Read the model definition and answer for the solid it produces. Units are mm, in the model's axes. Face numbers are marked on the shaded views. A direction names the side the tool comes from. Coordinates: 2 decimals unless noted, no trailing zeros. Write each loop counter-clockwise with the first axis right and the second up, starting at its lowest first coordinate (ties: lowest second). Pieces come first, ordered by that corner, then holes. Notation, with made-up numbers: (13.25, 12.5) -> (42.25, 12.5) arc R6 cw to (42.25, 21.5) -> close; hole circle Ø6 at (-13.5, -13.75). An arc over 180 degrees is marked (long way). Answer as a JSON object with one key per item and string values. Group by question number.
(1) Straight lines are drawn through the part: L1, parallel to Z at x = -51.4, y = -0.8; L2, parallel to X at y = -14, z = 2; L3, parallel to Z at x = 53, y = -2.5. For each, find the intervals that lie inside material, in ascending order.
(2) Flat-ended cylindrical pins translate along their axes: P1, Ø1, axis at x = -0.5, y = -8.5, coming from the -Z side; P2, Ø3, axis at x = -51.4, z = 8.2, coming from the -Y side; P3, Ø1.5, axis at x = 0, z = -8.2, coming from the +Y side. Find the tip coordinate at first contact, or state that the pin passes through.
(3) For a pull along X with two mould halves and no side action, classify the marked faces 1, 2, 3 and 4 as +X half, -X half, draft (parallel to the pull), parting line (faces both ways), or undercut.
(4) Find section A-A (x = 0). Give the vertices of the cut face in (y, z), then the cut area to 3 significant figures.
(5) Find section D-D (z = 0). Give the vertices of the cut face in (x, y).
(6) Find section B-B (y = -21.5). Give the vertices of the cut face in (x, z).
(7) Which of the six approach directions +Z, -Z, +X, -X, +Y, -Y give full straight-line access (tool end or side, diameter ignored) to the marked faces 5 and 6?
(8) Find section C-C (z = -8.2). Give the vertices of the cut face in (x, y).
from build123d import *

# Parameters (mm, degrees)
F0_W     = 124
F0_H     = 32
F0_R     = 1.25
F0_R_2   = 5.2
F0_R_3   = 4.95
F1_DEPTH = 3
F0_H_2   = 3
F2_DEPTH = 50
F5_DEPTH = 3
F6_DEPTH = 3


with BuildPart() as f1:
    # F0 (on Front) → F1 (new body)
    with BuildSketch(Plane.XZ):
        with Locations((0, 1)):
            Rectangle(F0_W, F0_H)
        with Locations((-51.4, -8.2)):
            Circle(F0_R, mode=Mode.SUBTRACT)
        with Locations((-51.4, 0)):
            Circle(F0_R_2, mode=Mode.SUBTRACT)
        with Locations((-8.2, 0)):
            Circle(F0_R, mode=Mode.SUBTRACT)
        with Locations((0, -8.2)):
            Circle(F0_R, mode=Mode.SUBTRACT)
        with Locations((51.4, -8.2)):
            Circle(F0_R, mode=Mode.SUBTRACT)
        Circle(F0_R_3, mode=Mode.SUBTRACT)
        with Locations((8.2, 0)):
            Circle(F0_R, mode=Mode.SUBTRACT)
        with Locations((51.4, 0)):
            Circle(F0_R_2, mode=Mode.SUBTRACT)
        with Locations((-51.4, 8.2)):
            Circle(F0_R, mode=Mode.SUBTRACT)
        with Locations((0, 8.2)):
            Circle(F0_R, mode=Mode.SUBTRACT)
        with Locations((51.4, 8.2)):
            Circle(F0_R, mode=Mode.SUBTRACT)
    extrude(amount=F1_DEPTH)

    # F0 (on Front) → F2 (join)
    with BuildSketch(Plane.XZ):
        with Locations((0, 18.5)):
            Rectangle(F0_W, F0_H_2)
    extrude(amount=F2_DEPTH)

    # F4 (on face) → F5 (join)
    with BuildSketch(Plane(origin=(-62, 0, 0), x_dir=(0, -1, 0), z_dir=(-1, 0, 0))):
        Polygon((3, 17), (3, -12), (40, 17), align=None)
    extrude(amount=-F5_DEPTH)

    # F3 (on face) → F6 (join)
    with BuildSketch(Plane.YZ.offset(62)):
        Polygon((-3, 17), (-40, 17), (-3, -12), align=None)
    extrude(amount=-F6_DEPTH)


solid = f1.part
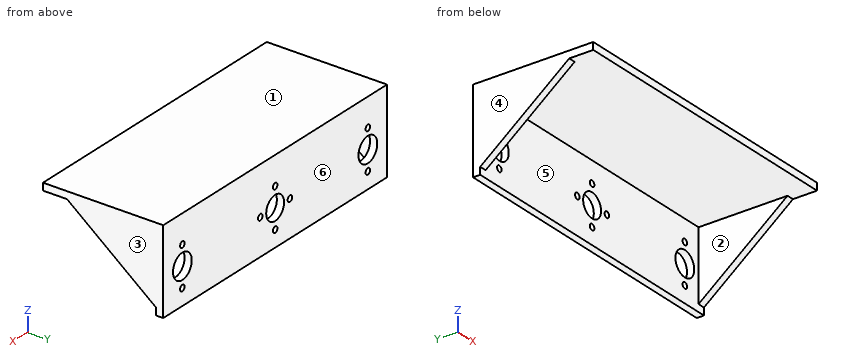
Results below:
{
 "1": {"L1": "z = -15 to -9.45, -6.95 to -5.2, 5.2 to 6.95, 9.45 to 20", "L2": "x = -62 to -59, 59 to 62", "L3": "z = -15 to -4.95, 4.95 to 20"},
 "2": {"P1": "stops at z = 17", "P2": "stops at y = -3", "P3": "passes through"},
 "3": {"face 1": "draft", "face 2": "undercut", "face 3": "+X half", "face 4": "-X half"},
 "4": {"outline": "(-50, 17) -> (-3, 17) -> (-3, 9.45) -> (0, 9.45) -> (0, 20) -> (-50, 20) -> close; (-3, -15) -> (0, -15) -> (0, -9.45) -> (-3, -9.45) -> close; (-3, -6.95) -> (0, -6.95) -> (0, -4.95) -> (-3, -4.95) -> close; (-3, 4.95) -> (0, 4.95) -> (0, 6.95) -> (-3, 6.95) -> close", "area": "201 mm2"},
 "5": {"outline": "(-62, -18.31) -> (-59, -18.31) -> (-59, -3) -> (-56.6, -3) -> (-56.6, 0) -> (-62, 0) -> close; (-46.2, -3) -> (-9.45, -3) -> (-9.45, 0) -> (-46.2, 0) -> close; (-6.95, -3) -> (-4.95, -3) -> (-4.95, 0) -> (-6.95, 0) -> close; (4.95, -3) -> (6.95, -3) -> (6.95, 0) -> (4.95, 0) -> close; (9.45, -3) -> (46.2, -3) -> (46.2, 0) -> (9.45, 0) -> close; (56.6, -3) -> (59, -3) -> (59, -18.31) -> (62, -18.31) -> (62, 0) -> (56.6, 0) -> close"},
 "6": {"outline": "(-62, 2.5) -> (-59, 2.5) -> (-59, 17) -> (59, 17) -> (59, 2.5) -> (62, 2.5) -> (62, 20) -> (-62, 20) -> close"},
 "7": {"face 5": "-Z, -Y", "face 6": "+Z, -Z, +X, -X, +Y"},
 "8": {"outline": "(-62, -7.85) -> (-59, -7.85) -> (-59, -3) -> (-52.65, -3) -> (-52.65, 0) -> (-62, 0) -> close; (-50.15, -3) -> (-1.25, -3) -> (-1.25, 0) -> (-50.15, 0) -> close; (1.25, -3) -> (50.15, -3) -> (50.15, 0) -> (1.25, 0) -> close; (52.65, -3) -> (59, -3) -> (59, -7.85) -> (62, -7.85) -> (62, 0) -> (52.65, 0) -> close"}
}
